```python
from build123d import *

# Parameters (mm, degrees)
SKETCH_1_W          = 29.5
SKETCH_1_H          = 12
EXTRUDE_1_DEPTH     = 23.4
SKETCH_3_W          = 23.5
SKETCH_3_H          = 12
CUT_EXTRUDE_1_DEPTH = 15
SKETCH_4_R          = 1.4
CUT_EXTRUDE_2_DEPTH = 39.12886046
FILLET_1_RADIUS     = 6
FILLET_1_LENGTH     = 3
MIRROR_START        = 11.75
MIRROR_1_DEPTH      = 3
HOLE_WIZARD_M5_1_D  = 5.3
CUT_EXTRUDE_4_DEPTH = 5


# Read off the part's stored shape, not the designer's step: 镜向1
with BuildPart() as part:
    # 草图1 → 凸台-拉伸1 (new body)
    with BuildSketch(Plane(origin=(0, 0, 0), x_dir=(1, 0, 0), z_dir=(0, 1, 0))):
        Rectangle(SKETCH_1_W, SKETCH_1_H)
    extrude(amount=EXTRUDE_1_DEPTH)

    # 草图3 → 切除-拉伸1 (cut)
    with BuildSketch(Plane(origin=(0, 23.4, 0), x_dir=(1, 0, 0), z_dir=(0, 1, 0))):
        Rectangle(SKETCH_3_W, SKETCH_3_H)
    extrude(amount=-CUT_EXTRUDE_1_DEPTH, mode=Mode.SUBTRACT)

    # 草图4 → 切除-拉伸2 (cut, through all)
    with BuildSketch(Plane.ZY.offset(14.75)):
        with Locations((0, 19)):
            Circle(SKETCH_4_R)
    extrude(amount=-CUT_EXTRUDE_2_DEPTH, mode=Mode.SUBTRACT)

    # 圆角1: full round fillet: the end face becomes a half cylinder, R = half its width
    fillet_1_face = Plane((-13.25, 23.4, 0), x_dir=(-1, 0, 0), z_dir=(0, 1, 0))  # on the end face: x along it, z out of the body
    fillet_1_slab = fillet_1_face.offset(-FILLET_1_RADIUS / 2) * Box(FILLET_1_LENGTH, 2 * FILLET_1_RADIUS, FILLET_1_RADIUS, mode=Mode.PRIVATE)  # the body's end, R deep
    fillet_1_round = Plane((-13.25, 17.4, 0), x_dir=(0, 1, 0), z_dir=(-1, 0, 0)) * Cylinder(FILLET_1_RADIUS, FILLET_1_LENGTH, mode=Mode.PRIVATE)  # its axis R under the face
    add(fillet_1_slab - fillet_1_round, mode=Mode.SUBTRACT)

    # 镜向1 outline → 镜向1 (cut)
    with BuildSketch(Plane.YZ.offset(MIRROR_START)):
        with BuildLine():
            Line((23.4, 6), (17.4, 6))
            ThreePointArc((17.4, 6), (21.642640687, 4.242640687), (23.4, 0))
            Line((23.4, 0), (23.4, 6))
        make_face()
        with BuildLine():
            Line((23.4, -6), (23.4, 0))
            ThreePointArc((23.4, 0), (21.642640687, -4.242640687), (17.4, -6))
            Line((17.4, -6), (23.4, -6))
        make_face()
    extrude(amount=MIRROR_1_DEPTH, mode=Mode.SUBTRACT)

    # M5 间隙孔1 (through all)
    with Locations(Plane(origin=(0, 0, 0), x_dir=(-1, 0, 0), z_dir=(0, -1, 0))):
        with Locations((-6.75, 0), (6.75, 0)):
            Hole(HOLE_WIZARD_M5_1_D / 2)

    # 草图10 → 切除-拉伸4 (cut)
    with BuildSketch(Plane.XZ.offset(-8.4)):
        Polygon((1.957992766, 0), (4.353996383, -4.15), (9.146003617, -4.15), (11.542007234, 0), (9.146003617, 4.15), (4.353996383, 4.15), align=None)
        Polygon((-11.542007234, 0), (-9.146003617, -4.15), (-4.353996383, -4.15), (-1.957992766, 0), (-4.353996383, 4.15), (-9.146003617, 4.15), align=None)
    extrude(amount=CUT_EXTRUDE_4_DEPTH, mode=Mode.SUBTRACT)


solid = part.part
```
Geometry: final body of the model. Coordinates: model frame, mm. A direction names the side the tool comes from. Round coordinates to 2 decimals unless told otherwise and drop trailing zeros. Write each loop counter-clockwise with the first axis right and the second up, starting at its lowest first coordinate (ties: lowest second). Pieces come first, ordered by that corner, then holes.
Item 1: Pin query (flat end, axial travel): P1, Ø6, axis at x = -2, z = -1.5, coming from the +Y side; P2, Ø2.5, axis at x = 7, z = -2, coming from the +Y side; P3, Ø1.7, axis at y = 19, z = 0, coming from the -X side. Return the tip coordinate at first contact, or that it passes through.
Item 2: Section query B-B (y = 2.25). Return loops of the section in (x, z), plus the area to 3 significant figures.
Item 3: Material intervals for L1, parallel to Z at x = 6, y = 4.25; L2, parallel to X at y = 13, z = 1.5; L3, parallel to Y at x = -6.75, z = -5.25, sorted ascending.
Item 4: Section query A-A (x = -6.75). Return loops of the section in (y, z).
Item 5: Section query D-D (z = 2). Return loops of the section in (x, y), plus the area to 3 significant figures.
Item 6: Mould query, pull axis X, two halves, no side actions, for faces 4 (the face through (-4.69, 3.4, 1.9)), 5 (the face through (14.75, 12, 0)), 6 (the face through (0, 5, -6)). Classes: +X half, -X half, draft (parallel to the pull), parting line (faces both ways), or undercut.
Item 7: Set-up query: faces 1 (the face through (-14.75, 12, 0)), 2 (the face through (-7, 6, 4.15)), 3 (the face through (0, 8.4, 0)). Return all of +Z, -Z, +X, -X, +Y, -Y with unobstructed straight access to the full face (end or side cutting, diameter ignored); none if empty.
Item 8: Section query C-C (y = 19.75). Return loops of the section in (x, z), plus the area to 3 significant figures.
Completed:
1. P1: stops at y = 8.4
1. P2: stops at y = 3.4
1. P3: passes through
2. outline: (-14.75, -6) - (14.75, -6) - (14.75, 6) - (-14.75, 6) - close; hole circle Ø5.3 at (-6.75, 0); hole circle Ø5.3 at (6.75, 0)
2. area: 310 mm2
3. L1: z = -6 to -4.15, 4.15 to 6
3. L2: x = -14.75 to -11.75, 11.75 to 14.75
3. L3: y = 0 to 8.4
4. outline: (0, -6) - (8.4, -6) - (8.4, -4.15) - (3.4, -4.15) - (3.4, -2.65) - (0, -2.65) - close; (0, 2.65) - (3.4, 2.65) - (3.4, 4.15) - (8.4, 4.15) - (8.4, 6) - (0, 6) - close
5. outline: (-14.75, 0) - (-8.49, 0) - (-8.49, 3.4) - (-10.39, 3.4) - (-10.39, 8.4) - (-11.75, 8.4) - (-11.75, 23.06) - (-14.75, 23.06) - close; (-5.01, 0) - (5.01, 0) - (5.01, 3.4) - (3.11, 3.4) - (3.11, 8.4) - (-3.11, 8.4) - (-3.11, 3.4) - (-5.01, 3.4) - close; (8.49, 0) - (14.75, 0) - (14.75, 23.06) - (11.75, 23.06) - (11.75, 8.4) - (10.39, 8.4) - (10.39, 3.4) - (8.49, 3.4) - close
5. area: 239 mm2
6. face 4: undercut
6. face 5: +X half
6. face 6: draft
7. face 1: +Z, -Z, -X, +Y, -Y
7. face 2: +Y
7. face 3: +Z, -Z, +Y
8. outline: (-14.75, -5.52) - (-11.75, -5.52) - (-11.75, -1.18) - (-14.75, -1.18) - close; (-14.75, 1.18) - (-11.75, 1.18) - (-11.75, 5.52) - (-14.75, 5.52) - close; (11.75, -5.52) - (14.75, -5.52) - (14.75, -1.18) - (11.75, -1.18) - close; (11.75, 1.18) - (14.75, 1.18) - (14.75, 5.52) - (11.75, 5.52) - close
8. area: 52.1 mm2
